Verification items for this drawing (mm, ordinates from the low corner). Round coordinates to 2 decimals unless told otherwise and drop trailing zeros. Loops run counter-clockwise (first coordinate to the right, second up) from the corner with the lowest first, then second, coordinate; pieces in that order, holes last. Notation, with made-up numbers: M -16.5,19 L 32.5,19 A28 ccw 32.5,56 Z; hole C 23,39.25 d10. An arc over 180 degrees is marked long. One line per item, written item: value.
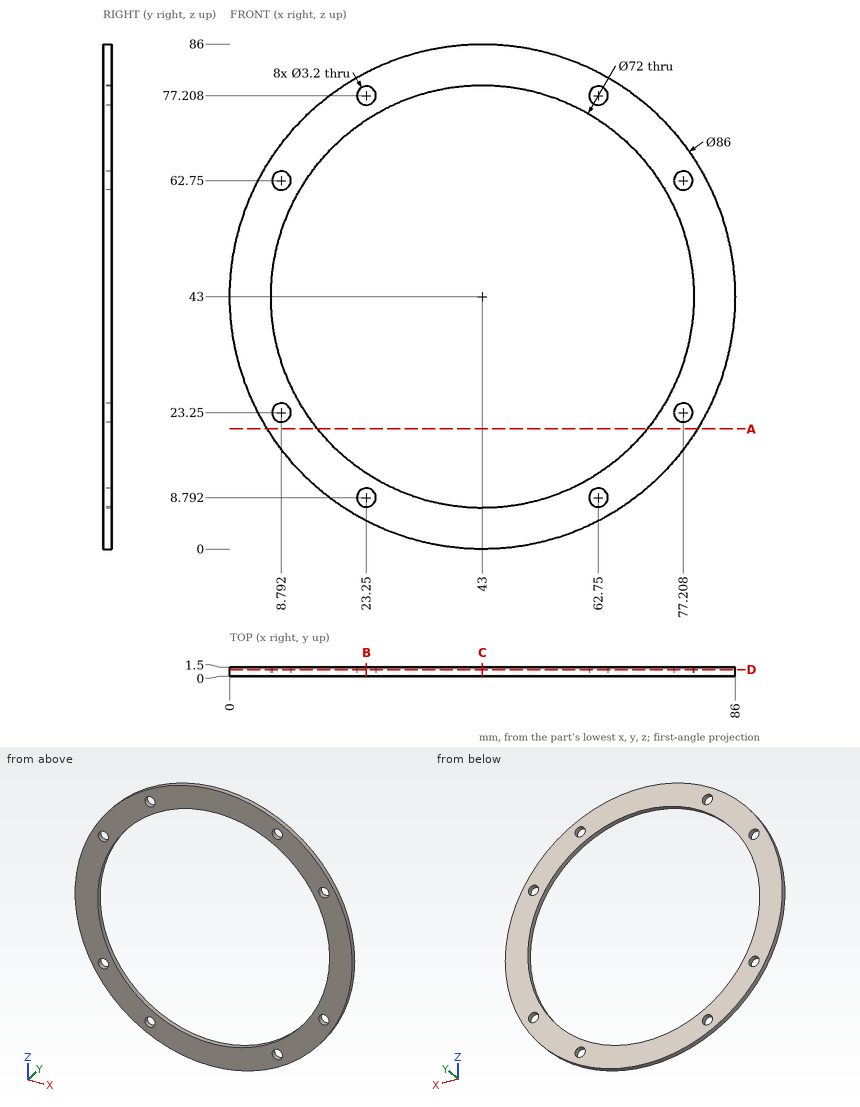
(1) Sectioned sample at B-B on x = 23.25. Enter the section's corners in (y, z).
Completed:
outline: M 0,4.8 L 1.5,4.8 L 1.5,7.19 L 0,7.19 Z; M 0,10.39 L 1.5,10.39 L 1.5,12.9 L 0,12.9 Z; M 0,73.1 L 1.5,73.1 L 1.5,75.61 L 0,75.61 Z; M 0,78.81 L 1.5,78.81 L 1.5,81.2 L 0,81.2 Z
(2) Sectioned sample at C-C on x = 43. Enter the section's corners in (y, z).
Completed:
outline: M 0,0 L 1.5,0 L 1.5,7 L 0,7 Z; M 0,79 L 1.5,79 L 1.5,86 L 0,86 Z
(3) Depth check by flat-ended pin: pin 1 Ø6 at (x, z) = (69, 27) entering from +Y. Enter the tip coordinate at first touch or a pass-through.
Completed:
pin 1: passes through
(4) Sectioned sample at D-D on y = 1.1. Count the separate pieces of the cut face and the enclosed holes in it, and give its area (3 significant figures).
Completed:
separate pieces: 1
enclosed holes: 9
area: 1,670 mm^2
(5) Sectioned sample at A-A on z = 20.5. Enter the section's corners in (x, y), and give its area (3 significant figures).
Completed:
outline: M 6.36,0 L 14.9,0 L 14.9,1.5 L 6.36,1.5 Z; M 71.1,0 L 79.64,0 L 79.64,1.5 L 71.1,1.5 Z
area: 25.6 mm^2
(6) Thickness scan on L1, parallel to Z at x = 23.25, y = 1.1; L2, parallel to X at y = 0.5, z = 23. Record the ranges inside material, lowest first. Write a range as from..to.
Completed:
L1: z = 4.8..7.19, 10.39..12.9, 73.1..75.61, 78.81..81.2
L2: x = 4.93..7.21, 10.37..13.07, 72.93..75.63, 78.79..81.07
